```python
from build123d import *

# Parameters (mm, degrees)
F1_DEPTH = 25.4
F2_R     = 6.963826
F3_DEPTH = 25.4
F5_DEPTH = 12.7


with BuildPart() as f1:
    # F0 (on Front) → F1 (new body)
    with BuildSketch(Plane.XZ):
        Polygon((0, 38.1), (0, 0), (69.85, 0), (69.85, 12.7), (25.4, 12.7), (25.4, 38.1), align=None)
    extrude(amount=F1_DEPTH)

    # F2 (on face) → F3 (cut)
    with BuildSketch(Plane.XZ.offset(25.4)):
        with Locations((12.7, 19.05)):
            Circle(F2_R)
        with BuildLine():
            ThreePointArc((0, 25.4), (12.7, 33.255156), (25.4, 25.4))
            Line((25.4, 25.4), (25.4, 38.1))
            Line((25.4, 38.1), (0, 38.1))
            Line((0, 38.1), (0, 25.4))
        make_face()
    extrude(amount=-F3_DEPTH, mode=Mode.SUBTRACT)

    # F4 (on Top) → F5 (cut)
    with BuildSketch(Plane.XY):
        with BuildLine():
            ThreePointArc((47.063009, -12.219809), (45.820597, -15.790974), (42.629922, -17.819863))
            Line((42.629922, -17.819863), (55.326719, -17.534672))
            ThreePointArc((55.326719, -17.534672), (49.649912, -12.184477), (54.918351, -6.431715))
            Line((54.918351, -6.431715), (43.04726, -6.734904))
            ThreePointArc((43.04726, -6.734904), (45.951759, -8.820897), (47.063009, -12.219809))
        make_face()
        with BuildLine():
            ThreePointArc((54.918351, -6.431715), (49.649912, -12.184477), (55.326719, -17.534672))
            ThreePointArc((55.326719, -17.534672), (59.174368, -15.864457), (60.757759, -11.980272))
            ThreePointArc((60.757759, -11.980272), (59.130503, -8.051728), (55.201958, -6.424471))
            Line((55.201958, -6.424471), (54.918351, -6.431715))
        make_face()
        with BuildLine():
            Line((43.04726, -6.734904), (39.293736, -6.83077))
            ThreePointArc((39.293736, -6.83077), (35.803833, -13.891235), (42.629922, -17.819863))
            ThreePointArc((42.629922, -17.819863), (45.820597, -15.790974), (47.063009, -12.219809))
            ThreePointArc((47.063009, -12.219809), (45.951759, -8.820897), (43.04726, -6.734904))
        make_face()
    extrude(amount=F5_DEPTH, mode=Mode.SUBTRACT)


solid = f1.part
```
The model under review builds one solid part; all positions refer to its coordinate system, in mm. A direction names the side the tool comes from. Round coordinates to 2 decimals unless told otherwise and drop trailing zeros. Loops run counter-clockwise (first coordinate to the right, second up) from the corner with the lowest first, then second, coordinate; pieces in that order, holes last. Notation, with made-up numbers: (-27, 2.25) - (21, 2.25) arc R25 cw to (21, 21.25) - close; hole circle Ø7 at (79, 65). An arc over 180 degrees is marked (long way). Write each question's results on one line, items separated by ' | '. Start each with the question number.
Q1. Take a section at B-B on x = 12.7. Give the boundary of the cut face in (y, z).
Q2. Tool access review of faces 1 (the flat face through (25.4, -13, 19)), 2 (the cylindrical face through (12.48, -12.878, 33.253)): name each direction out of +Z, -Z, +X, -X, +Y, -Y from which nothing blocks a thin tool from reaching the whole face with its end or side.
Q3. Draft analysis for pull direction Y (two halves, no side actions). For faces 3 (the cylindrical face through (35.77, -13.77, 6.26)), 4 (the flat face through (27, 0, 9)), 5 (the flat face through (69.85, -13, 6)), 6 (the flat face through (27, -25.4, 9)), state which applies: pulls with the +Y half, pulls with the -Y half, needs draft (parallel to the pull), parting line crosses it, or undercut.
Q4. Wall thickness on line 1 along Z through (x, y) = (12.7, -7.25); line 2 along X through (y, z) = (-20.25, 19.5); line 3 along Z through (x, y) = (15, -18.5): over which ranges is each line inside the solid? List them lowest first. Write a range as [from, to].
Q5. Take a section at A-A on z = 19.05. Give the boundary of the cut face in (x, y).
Q6. Insertion check: P1, Ø1, axis at x = 14.5, y = -20, coming from the +Z side; P2, Ø4, axis at x = 44, y = -21, coming from the +Z side; P3, Ø14, axis at y = -13.5, z = 19, coming from the +X side. Each pin has a flat end and moves straight along its axis. Give the tip position at first contact, or say it passes through.
Q7. Take a section at C-C on y = -14. Give the boundary of the cut face in (x, z).
Q8. Take a section at D-D on z = 4. Give the boundary of the cut face in (x, y).
Data:
1) outline: (-25.4, 0) - (0, 0) - (0, 12.09) - (-25.4, 12.09) - close; (-25.4, 26.01) - (0, 26.01) - (0, 33.26) - (-25.4, 33.26) - close
2) face 1: +Z, +X, +Y, -Y | face 2: +Z, +Y, -Y
3) face 3: undercut | face 4: pulls with the +Y half | face 5: needs draft | face 6: pulls with the -Y half
4) line 1: z = [0, 12.09], [26.01, 33.26] | line 2: x = [0, 5.75], [19.65, 25.4] | line 3: z = [0, 12.48], [25.62, 33.07]
5) outline: (0, -25.4) - (5.74, -25.4) - (5.74, 0) - (0, 0) - close; (19.66, -25.4) - (25.4, -25.4) - (25.4, 0) - (19.66, 0) - close
6) P1: stops at z = 33.2 | P2: stops at z = 12.7 | P3: stops at x = 69.85
7) outline: (0, 0) - (35.84, 0) - (35.84, 12.7) - (25.4, 12.7) - (25.4, 25.4) arc R14.19 ccw to (0, 25.4) - close; (60.38, 0) - (69.85, 0) - (69.85, 12.7) - (60.38, 12.7) - close; hole circle Ø13.93 at (12.7, 19.05)
8) outline: (0, -25.4) - (69.85, -25.4) - (69.85, 0) - (0, 0) - close; hole (39.29, -6.83) arc R5.75 ccw to (42.63, -17.82) - (55.33, -17.53) arc R5.56 ccw to (60.76, -11.98) arc R5.56 ccw to (55.2, -6.42) - (54.92, -6.43) - (43.05, -6.73) - close
